Autodesk Inventor part; units mm, degrees
ref_plane "YZ Plane" through (0, 0, 0) normal (1, 0, 0) x (0, 1, 0)
ref_plane "XZ Plane" through (0, 0, 0) normal (0, 1, 0) x (-1, 0, 0)
ref_plane "XY Plane" through (0, 0, 0) normal (0, 0, 1) x (1, 0, 0)
sketch "Sketch1" plane through (0, 0, 0) normal (0, 0, 1) x (1, 0, 0)
  line L0 (-10, -10) -> (10, -10)
  line L1 (10, -10) -> (10, 10)
  line L2 (10, 10) -> (-10, 10)
  line L3 (-10, 10) -> (-10, -10)
  line L4 (-10, -10) -> (10, 10) construction
  line L5 (10, -10) -> (-10, 10) construction
  point P0 (0, 0)
  dimension "d0" = 20
  dimension "d1" = 20
extrude "Extrusion1" add sketch "Sketch1" along normal blind 4
sketch "Sketch2" plane through (0, 0, 4) normal (0, 0, 1) x (1, 0, 0)
  line L0 (-10.25, 10.25) -> (10.25, 10.25)
  line L1 (10.25, 10.25) -> (10.25, -10.25)
  line L2 (10.25, -10.25) -> (-10.25, -10.25)
  line L3 (-10.25, -10.25) -> (-10.25, 10.25)
  line L4 (-10.25, 10.25) -> (10.25, -10.25) construction
  line L5 (10.25, 10.25) -> (-10.25, -10.25) construction
  point P0 (0, 0)
  dimension "d4" = 20.5
  dimension "d5" = 20.5
extrude "Extrusion2" add sketch "Sketch2" along normal blind 2.5
fillet "Fillet1" radius 6 8 edges at (-10, 10, 2) (10, 10, 2) (-10, -10, 2) (-10.25, -10.25, 5.25) (-10.25, 10.25, 5.25) (10.25, 10.25, 5.25) (10, -10, 2) (10.25, -10.25, 5.25)
sketch "Sketch3" plane through (0, 0, 4) normal (0, 0, -1) x (-1, 0, 0)
  line L0 (-4.25, 10.25) -> (4.25, 10.25)
  line L1 (2.5, 9.75) -> (-2.5, 9.75)
  line L2 (-2.5, 9.75) -> (-2.5, 10.25)
  line L3 (-2.5, 10.25) -> (2.5, 10.25)
  line L4 (2.5, 10.25) -> (2.5, 9.75)
  line L5 (-4, 10) -> (4, 10)
  line L6 (2.5, 9.75) -> (-2.5, 10.25) construction
  line L7 (-2.5, 9.75) -> (2.5, 10.25) construction
  point P0 (0, 0)
  point P1 (0, 10)
  dimension "d9" = 5
extrude "Extrusion3" add sketch "Sketch3" along normal blind 1
sketch "Sketch4" plane through (0, 0, 6.5) normal (0, 0, 1) x (1, 0, 0)
  circle A0 centre (0, 0) radius 7
  line L0 (-6, -1.25) -> (6, -1.25)
  line L1 (6, -1.25) -> (6, 1.25)
  line L2 (6, 1.25) -> (-6, 1.25)
  line L3 (-6, 1.25) -> (-6, -1.25)
  line L4 (-6, -1.25) -> (6, 1.25) construction
  line L5 (6, -1.25) -> (-6, 1.25) construction
  line L6 (1.25, -6) -> (-1.25, -6)
  line L7 (-1.25, -6) -> (-1.25, 6)
  line L8 (-1.25, 6) -> (1.25, 6)
  line L9 (1.25, 6) -> (1.25, -6)
  line L10 (1.25, -6) -> (-1.25, 6) construction
  line L11 (-1.25, -6) -> (1.25, 6) construction
  point P0 (-1.25, 1.25)
  point P1 (1.25, 1.25)
  point P2 (1.25, -1.25)
  point P3 (-1.25, -1.25)
  dimension "d12" = 14
  dimension "d13" = 12
  dimension "d14" = 2.5
  dimension "d15" = 2.5
  dimension "d16" = 12
extrude "Extrusion4" cut sketch "Sketch4" against normal blind 0.5
equation "\"d1\" = d0"
equation "\"d5\" = d4"
properties part number "Health-Item-Pack"
Input: part model. Units: mm. Frame: model coordinates. A direction names the side the tool comes from. Round coordinates to 2 decimals unless told otherwise and drop trailing zeros. Loops run counter-clockwise (first coordinate to the right, second up) from the corner with the lowest first, then second, coordinate; pieces in that order, holes last.
1) Set-up query: faces 1 (the cylindrical face through (6.466, -2.681, 6.254)), 2 (the flat face through (-10, 0, 2)), 3 (the cylindrical face through (8.196, -8.289, 2.028)), 4 (the flat face through (0, -10, 2)). Return all of +Z, -Z, +X, -X, +Y, -Y with unobstructed straight access to the full face (end or side cutting, diameter ignored); none if empty.
Ans:
face 1: +Z
face 2: -Z, -X, +Y, -Y
face 3: -Z, +X, -Y
face 4: -Z, +X, -X, -Y
2) Material intervals for line 1 (Y direction, x = 0, z = 6.4); line 2 (X direction, y = 5, z = 6.25); line 3 (Z direction, x = 3.5, y = 3.25), sorted ascending.
Ans:
line 1: y = -10.25 to -7, -6 to 6, 7 to 10.25
line 2: x = -10.2 to -4.9, -1.25 to 1.25, 4.9 to 10.2
line 3: z = 0 to 6
3) Section query D-D on z = 1. Return the cut outline in (x, y), plus the area to 3 significant figures.
Ans:
outline: (-10, -4) arc R6 ccw to (-4, -10) - (4, -10) arc R6 ccw to (10, -4) - (10, 4) arc R6 ccw to (4, 10) - (-4, 10) arc R6 ccw to (-10, 4) - close
area: 369 mm2
4) Pin query (flat end, axial travel): pin 1 (3 mm diameter, centred on y = 1.5, z = 1.5, fed in from +X); pin 2 (3 mm diameter, centred on y = 8, z = 5.5, fed in from +X); pin 3 (1.5 mm diameter, centred on x = 3.5, y = 5, fed in from +Z); pin 4 (12 mm diameter, centred on x = -6, y = 5, fed in from -Z). Return the tip coordinate at first contact, or that it passes through.
Ans:
pin 1: stops at x = 10
pin 2: stops at x = 9.81
pin 3: stops at z = 6
pin 4: stops at z = 0
5) Section query C-C on y = 0. Return the cut outline in (x, z).
Ans:
outline: (-10.25, 4) - (-10, 4) - (-10, 0) - (10, 0) - (10, 4) - (10.25, 4) - (10.25, 6.5) - (7, 6.5) - (7, 6) - (6, 6) - (6, 6.5) - (-6, 6.5) - (-6, 6) - (-7, 6) - (-7, 6.5) - (-10.25, 6.5) - close
6) Pull-direction query (X, two-part tool) for faces 5 (the flat face through (1.5, -1.5, 6)), 6 (the flat face through (0, 0, 6.5)), 7 (the cylindrical face through (-8.539, -8.446, 5.268)); classes: released by +X, released by -X, zero draft, split by the parting line, or undercut.
Ans:
face 5: undercut
face 6: zero draft
face 7: released by -X
7) Section query B-B on x = 0. Return the cut outline in (y, z), plus the area to 4 significant figures.
Ans:
outline: (-10.25, 4) - (-10, 4) - (-10, 0) - (10, 0) - (10, 3) - (10.25, 3) - (10.25, 6.5) - (7, 6.5) - (7, 6) - (6, 6) - (6, 6.5) - (-6, 6.5) - (-6, 6) - (-7, 6) - (-7, 6.5) - (-10.25, 6.5) - close
area: 130.5 mm2
8) Section query A-A on z = 3.25. Return the cut outline in (x, y), plus the area to 3 significant figures.
Ans:
outline: (-10, -4) arc R6 ccw to (-4, -10) - (4, -10) arc R6 ccw to (10, -4) - (10, 4) arc R6 ccw to (4, 10) - (2.5, 10) - (2.5, 10.25) - (-2.5, 10.25) - (-2.5, 10) - (-4, 10) arc R6 ccw to (-10, 4) - close
area: 370 mm2
